Read the model definition and answer for the solid it produces. Units are mm, in the model's axes. A direction names the side the tool comes from. Give positions to 0.01 mm unless a question says otherwise; leave off trailing zeros. Order: outer loops, then holes, each group sorted by start corner. A loop starts at its lowest first (then second) coordinate and runs counter-clockwise, first axis right, second up. Notation, with made-up numbers: (79, 65.25) - (87, 65.25) arc R17 ccw to (87, 78.25) - close; hole circle Ø8 at (18, 80). An arc over 180 degrees is marked (long way). Use a Markdown table: item, result. Add a question column.
1. A cutting plane is placed at A-A on y = 4.25. State how many separate pieces and enclosed holes the cut face has, and give its area (3 significant figures).
2. For a pull along Z with two mould halves and no side action, classify faces 1 (the cylindrical face through (42.074, 7.624, -19.404)), 2 (the flat face through (-7.5, 4, 20)), 3 (the flat face through (-34, 1, -1)), 4 (the cylindrical face through (44.1, 4.68, 24.14)) as released by +Z, released by -Z, zero draft, split by the parting line, or undercut.
3. A cutting plane is placed at C-C on x = 28.5. Determine the outline of the cut face in (y, z), and give its area (3 significant figures).
4. A cutting plane is placed at B-B on x = -39. Determine the outline of the cut face in (y, z).
5. Flat-ended cylindrical pins translate along their axes: P1, Ø3.5, axis at x = 26, z = 16.5, coming from the -Y side; P2, Ø5, axis at x = -27.5, y = 3.5, coming from the +Z side; P3, Ø0.8, axis at x = -25, y = 0.5, coming from the +Z side. Find the tip coordinate at first contact, or state that the pin passes through.
6. Which of the six approach directions +Z, -Z, +X, -X, +Y, -Y give full straight-line access (tool end or side, diameter ignored) to faces 5 (the flat face through (39, 1, -8)), 6 (the flat face through (6.4, 1.3, -19)), 7 (the cylindrical face through (42.074, 7.624, 18.596)), 8 (the flat face through (-40, 4, -7.5)), 9 (the flat face through (0, 1, 14))?
7. A cutting plane is placed at D-D on z = 2.5. Determine the outline of the cut face in (x, y), and give its area (3 significant figures).
8. Consider L1, parallel to Z at x = -39, y = 2.1; L2, parallel to X at y = 5, z = 17; L3, parallel to X at y = 6.85, z = -19. Determine where each line is inside the solid, lowest interval first.
```python
from build123d import *

# Parameters (mm, degrees)
SKETCH_1_R          = 1.6
EXTRUDE_1_DEPTH     = 8.5
CUT_EXTRUDE_START   = -8.5
SKETCH_2_W          = 15
SKETCH_2_H          = 10.3
SKETCH_2_W_2        = 10.3
SKETCH_2_H_2        = 15
CUT_EXTRUDE_1_DEPTH = 6.5
SKETCH_3_W          = 9.2
SKETCH_3_H          = 7.6
CUT_EXTRUDE_2_DEPTH = 3.4
SKETCH_4_W          = 8
SKETCH_4_H          = 6
CUT_EXTRUDE_3_DEPTH = 2.6
SKETCH_7_W          = 9.6
SKETCH_7_H          = 11.1
CUT_EXTRUDE_4_DEPTH = 1
SKETCH_8_W          = 12.3
SKETCH_8_H          = 5.7
CUT_EXTRUDE_5_DEPTH = 3.4
SKETCH_8_3_W        = 14.7
SKETCH_8_3_H        = 12.8
CUT_EXTRUDE_6_DEPTH = 2
SKETCH_8_4_W        = 11.8
SKETCH_8_4_H        = 18.9
SKETCH_8_4_W_2      = 4.2
SKETCH_8_4_H_2      = 2
SKETCH_8_4_W_3      = 8.3
SKETCH_8_4_H_3      = 1.4
SKETCH_8_4_W_4      = 1.2
SKETCH_8_4_W_5      = 3.4
SKETCH_8_4_W_6      = 18.9
SKETCH_8_4_H_4      = 11.8
CUT_EXTRUDE_7_DEPTH = 1
SKETCH_9_R          = 3.1
CUT_EXTRUDE_8_DEPTH = 2.7
SKETCH_10_R         = 3.1
EXTRUDE_2_DEPTH     = 1


with BuildPart() as part:
    # 草图1 → 凸台-拉伸1 (new body)
    with BuildSketch(Plane(origin=(0, 0, 0), x_dir=(1, 0, 0), z_dir=(0, 1, 0))):
        with BuildLine():
            Line((-42, -25), (42, -25))
            ThreePointArc((42, -25), (44.121320344, -24.121320344), (45, -22))
            Line((45, -22), (45, 22))
            ThreePointArc((45, 22), (44.121320344, 24.121320344), (42, 25))
            Line((42, 25), (-42, 25))
            ThreePointArc((-42, 25), (-44.121320344, 24.121320344), (-45, 22))
            Line((-45, 22), (-45, -22))
            ThreePointArc((-45, -22), (-44.121320344, -24.121320344), (-42, -25))
        make_face()
        with Locations(Location((-39, 19, 0), (0, 0, 270))):
            Circle(SKETCH_1_R, mode=Mode.SUBTRACT)
        with Locations(Location((39, 19, 0), (0, 0, 270))):
            Circle(SKETCH_1_R, mode=Mode.SUBTRACT)
        with Locations(Location((-39, -19, 0), (0, 0, 270))):
            Circle(SKETCH_1_R, mode=Mode.SUBTRACT)
        with Locations(Location((39, -19, 0), (0, 0, 270))):
            Circle(SKETCH_1_R, mode=Mode.SUBTRACT)
    extrude(amount=EXTRUDE_1_DEPTH)

    # 草图2 → 切除-拉伸1 (cut)
    with BuildSketch(Plane(origin=(0, 8.5, 0), x_dir=(1, 0, 0), z_dir=(0, 1, 0)).offset(CUT_EXTRUDE_START)):
        with Locations((0, -19.85)):
            Rectangle(SKETCH_2_W, SKETCH_2_H)
        with Locations((-25, -19.85)):
            Rectangle(SKETCH_2_W, SKETCH_2_H)
        with Locations((25, -19.85)):
            Rectangle(SKETCH_2_W, SKETCH_2_H)
        with Locations((-39.85, 0)):
            Rectangle(SKETCH_2_W_2, SKETCH_2_H_2)
        with Locations((39.85, 0)):
            Rectangle(SKETCH_2_W_2, SKETCH_2_H_2)
    extrude(amount=CUT_EXTRUDE_1_DEPTH, mode=Mode.SUBTRACT)

    # 草图3 → 切除-拉伸2 (cut)
    with BuildSketch(Plane(origin=(0, 8.5, 0), x_dir=(1, 0, 0), z_dir=(0, 1, 0)).offset(CUT_EXTRUDE_START)):
        with Locations((-9.142, 21.2)):
            Rectangle(SKETCH_3_W, SKETCH_3_H)
    extrude(amount=CUT_EXTRUDE_2_DEPTH, mode=Mode.SUBTRACT)

    # 草图4 → 切除-拉伸3 (cut)
    with BuildSketch(Plane(origin=(0, 8.5, 0), x_dir=(1, 0, 0), z_dir=(0, 1, 0)).offset(CUT_EXTRUDE_START)):
        with Locations((6.466, 22)):
            Rectangle(SKETCH_4_W, SKETCH_4_H)
    extrude(amount=CUT_EXTRUDE_3_DEPTH, mode=Mode.SUBTRACT)

    # 草图7 → 切除-拉伸4 (cut)
    with BuildSketch(Plane(origin=(0, 8.5, 0), x_dir=(1, 0, 0), z_dir=(0, 1, 0)).offset(CUT_EXTRUDE_START)):
        with Locations((-25, 27.45)):
            Rectangle(SKETCH_7_W, SKETCH_7_H)
    extrude(amount=CUT_EXTRUDE_4_DEPTH, mode=Mode.SUBTRACT)

    # 草图8 → 切除-拉伸5 (cut)
    with BuildSketch(Plane.XZ):
        with Locations((25, -22.15)):
            Rectangle(SKETCH_8_W, SKETCH_8_H)
    extrude(amount=-CUT_EXTRUDE_5_DEPTH, mode=Mode.SUBTRACT)

    # 草图8<3> → 切除-拉伸6 (cut)
    with BuildSketch(Plane.XZ):
        with Locations((27.35, 0)):
            Rectangle(SKETCH_8_3_W, SKETCH_8_3_H)
    extrude(amount=-CUT_EXTRUDE_6_DEPTH, mode=Mode.SUBTRACT)

    # 草图8<4> → 切除-拉伸7 (cut)
    with BuildSketch(Plane.XZ):
        with Locations((-39.1, 0)):
            Rectangle(SKETCH_8_4_W, SKETCH_8_4_H)
        with Locations((-29.4, 0)):
            Rectangle(SKETCH_8_4_W_2, SKETCH_8_4_H_2)
        with Locations((-25, -21.2)):
            Rectangle(SKETCH_8_4_W_3, SKETCH_8_4_H_3)
        with Locations((-17.06, -18.4)):
            Rectangle(SKETCH_8_4_W_4, SKETCH_8_4_H_2)
        with Locations((-1.312, -18.4)):
            Rectangle(SKETCH_8_4_W_4, SKETCH_8_4_H_2)
        with Locations((6.466, -18.3)):
            Rectangle(SKETCH_8_4_W_5, SKETCH_8_4_H_3)
        with Locations((39.1, 0)):
            Rectangle(SKETCH_8_4_W, SKETCH_8_4_H)
        with Locations((-25, 19.1)):
            Rectangle(SKETCH_8_4_W_6, SKETCH_8_4_H_4)
        with Locations((0, 19.1)):
            Rectangle(SKETCH_8_4_W_6, SKETCH_8_4_H_4)
        with Locations((25, 19.1)):
            Rectangle(SKETCH_8_4_W_6, SKETCH_8_4_H_4)
    extrude(amount=-CUT_EXTRUDE_7_DEPTH, mode=Mode.SUBTRACT)

    # 草图9 → 切除-拉伸8 (cut)
    with BuildSketch(Plane(origin=(0, 8.5, 0), x_dir=(1, 0, 0), z_dir=(0, 1, 0))):
        with Locations(Location((-39, 19, 0), (0, 0, 270))):
            Circle(SKETCH_9_R)
        with Locations(Location((-39, -19, 0), (0, 0, 270))):
            Circle(SKETCH_9_R)
        with Locations(Location((39, 19, 0), (0, 0, 270))):
            Circle(SKETCH_9_R)
        with Locations(Location((39, -19, 0), (0, 0, 270))):
            Circle(SKETCH_9_R)
    extrude(amount=-CUT_EXTRUDE_8_DEPTH, mode=Mode.SUBTRACT)

    # 草图10 → 凸台-拉伸2 (add)
    with BuildSketch(Plane(origin=(0, 8.5, 0), x_dir=(1, 0, 0), z_dir=(0, 1, 0))):
        with BuildLine():
            Line((-42, -25), (42, -25))
            ThreePointArc((42, -25), (44.121320344, -24.121320344), (45, -22))
            Line((45, -22), (45, 22))
            ThreePointArc((45, 22), (44.121320344, 24.121320344), (42, 25))
            Line((42, 25), (-42, 25))
            ThreePointArc((-42, 25), (-44.121320344, 24.121320344), (-45, 22))
            Line((-45, 22), (-45, -22))
            ThreePointArc((-45, -22), (-44.121320344, -24.121320344), (-42, -25))
        make_face()
        with Locations(Location((39, -19, 0), (0, 0, 270))):
            Circle(SKETCH_10_R, mode=Mode.SUBTRACT)
        with Locations(Location((39, 19, 0), (0, 0, 270))):
            Circle(SKETCH_10_R, mode=Mode.SUBTRACT)
        with Locations(Location((-39, -19, 0), (0, 0, 270))):
            Circle(SKETCH_10_R, mode=Mode.SUBTRACT)
        with Locations(Location((-39, 19, 0), (0, 0, 270))):
            Circle(SKETCH_10_R, mode=Mode.SUBTRACT)
    extrude(amount=EXTRUDE_2_DEPTH)


solid = part.part
```
Output values:
| question | item | result |
|---|---|---|
| 1 | separate pieces | 1 |
| 1 | enclosed holes | 4 |
| 1 | area | 3,690 mm² |
| 2 | face 1 | undercut |
| 2 | face 2 | zero draft |
| 2 | face 3 | undercut |
| 2 | face 4 | released by +Z |
| 3 | outline | (0, -19.3) - (3.4, -19.3) - (3.4, -25) - (9.5, -25) - (9.5, 25) - (6.5, 25) - (6.5, 14.7) - (1, 14.7) - (1, 13.2) - (0, 13.2) - (0, 6.4) - (2, 6.4) - (2, -6.4) - (0, -6.4) - close |
| 3 | area | 362 mm² |
| 4 | outline | (0, -25) - (9.5, -25) - (9.5, -22.1) - (5.8, -22.1) - (5.8, -20.6) - (0, -20.6) - close; (0, -17.4) - (5.8, -17.4) - (5.8, -15.9) - (9.5, -15.9) - (9.5, 15.9) - (5.8, 15.9) - (5.8, 17.4) - (0, 17.4) - (0, 9.45) - (1, 9.45) - (1, 7.5) - (6.5, 7.5) - (6.5, -7.5) - (1, -7.5) - (1, -9.45) - (0, -9.45) - close; (0, 20.6) - (5.8, 20.6) - (5.8, 22.1) - (9.5, 22.1) - (9.5, 25) - (0, 25) - close |
| 5 | P1 | y = 6.5 |
| 5 | P2 | z = 14.7 |
| 5 | P3 | z = 13.2 |
| 6 | face 5 | +X, -Y |
| 6 | face 6 | -Z, -Y |
| 6 | face 7 | +Y |
| 6 | face 8 | -X, -Y |
| 6 | face 9 | +Z, -Y |
| 7 | outline | (-45, 6.5) - (-34.7, 6.5) - (-34.7, 1) - (-33.2, 1) - (-33.2, 0) - (20, 0) - (20, 2) - (34.7, 2) - (34.7, 6.5) - (45, 6.5) - (45, 9.5) - (-45, 9.5) - close |
| 7 | area | 690 mm² |
| 8 | L1 | -25 to -20.6, -17.4 to -7.5, 7.5 to 17.4, 20.6 to 25 |
| 8 | L2 | -45 to -32.5, -17.5 to -7.5, 7.5 to 17.5, 32.5 to 45 |
| 8 | L3 | -45 to -42.1, -35.9 to 35.9, 42.1 to 45 |
